Autodesk Inventor part; units mm, degrees
ref_plane "YZ Plane" through (0, 0, 0) normal (1, 0, 0) x (0, 1, 0)
ref_plane "XZ Plane" through (0, 0, 0) normal (0, 1, 0) x (-1, 0, 0)
ref_plane "XY Plane" through (0, 0, 0) normal (0, 0, 1) x (1, 0, 0)
sketch "Sketch1" plane through (0, 0, 0) normal (1, 0, 0) x (0, 1, 0)
  line L0 (90, 90) -> (-90, 90)
  line L1 (-90, 90) -> (-90, -90)
  line L2 (-90, -90) -> (90, -90)
  line L3 (90, -90) -> (90, 90)
  line L4 (91, 91) -> (-91, 91)
  line L5 (-91, 91) -> (-91, -91)
  line L6 (-91, -91) -> (91, -91)
  line L7 (91, -91) -> (91, 91)
  point P0 (0, 0)
  dimension "d0" = 180
  dimension "d1" = 180
  dimension "d2" = 90
  dimension "d3" = 90
  dimension "d4" = 1
  dimension "d5" = 1
  dimension "d6" = 1
  dimension "d7" = 1
extrude "Extrusion1" add sketch "Sketch1" along normal blind 10
properties part number "frame"
The listing builds one solid part. Answer for the finished solid, in the listing's coordinates (mm). A direction names the side the tool comes from. Give positions to 0.01 mm unless a question says otherwise; leave off trailing zeros. Write each loop counter-clockwise with the first axis right and the second up, starting at its lowest first coordinate (ties: lowest second). Pieces come first, ordered by that corner, then holes. Notation, with made-up numbers: (-13, 35.5) - (45, 35.5) arc R15 cw to (45, 53.5) - close; hole circle Ø6 at (8.25, 58). An arc over 180 degrees is marked (long way). Use one line per item in the form item = value. Start each with the question number.
1) Consider line 1 along Z through (x, y) = (6, 63). Determine where the line is inside the solid, lowest interval first. Write a range as from..to.
2) Find section A-A on z = -47. Determine the outline of the cut face in (x, y).
3) Find section B-B on x = 4.25. Determine the outline of the cut face in (y, z).
4) The mould has two halves that part along Y. Classify faces 3 (the face through (5, 91, -1)), 4 (the face through (5, -90, 1)), 5 (the face through (5, -1, -91)): pulls with the +Y half, pulls with the -Y half, needs draft (parallel to the pull), parting line crosses it, or undercut.
5) A tool of negligible diameter and unlimited length cuts with its end or side. For faces 1 (the face through (5, -1, -90)), 2 (the face through (5, 1, 91)), from which of +Z, -Z, +X, -X, +Y, -Y can it reach the whole face along a straight path? Write none if from no direction.
Geometry results:
q1.line_1 = -91..-90, 90..91
q2.outline = (0, -91) - (10, -91) - (10, -90) - (0, -90) - close; (0, 90) - (10, 90) - (10, 91) - (0, 91) - close
q3.outline = (-91, -91) - (91, -91) - (91, 91) - (-91, 91) - close; hole (-90, -90) - (90, -90) - (90, 90) - (-90, 90) - close
q4.face_3 = pulls with the +Y half
q4.face_4 = undercut
q4.face_5 = needs draft
q5.face_1 = +X, -X
q5.face_2 = +Z, +X, -X, +Y, -Y
